```python
from build123d import *

# Parameters (mm, degrees)
F1_R     = 43.202069
F2_DEPTH = 60.706


with BuildPart() as f2:
    # F1 (on face) → F2 (new body)
    with BuildSketch(Plane.YZ):
        Circle(F1_R)
        Polygon((-6.760658, 25.522216), (22.183912, 14.316566), (20.471069, -16.674092), (-9.532095, -24.621722), (-26.362228, 1.457031), align=None, mode=Mode.SUBTRACT)
    extrude(amount=F2_DEPTH)


solid = f2.part
```
Source: CAD feature listing. Evaluate the final solid. Frame: model axes, mm. A direction names the side the tool comes from. Give positions to 0.01 mm unless a question says otherwise; leave off trailing zeros. Write each loop counter-clockwise with the first axis right and the second up, starting at its lowest first coordinate (ties: lowest second). Pieces come first, ordered by that corner, then holes.
1. Access query for faces 1 (the face through (29.928, 5.68, -20.592)), 2 (the face through (0, -20, -9)). Directions: +Z, -Z, +X, -X, +Y, -Y. A direction counts if a zero-diameter tool reaches every point of the face in a straight line with its end or side. Return the directions, or none.
2. Section query B-B (y = 16.5). Return the cut outline in (x, z).
3. Section query C-C (z = 0). Return the cut outline in (x, y).
4. Section query A-A (x = 22). Return the cut outline in (y, z), then the cut area to 3 significant figures.
5. Section query D-D (y = 28). Return the cut outline in (x, z), then the cut area to 3 significant figures.
6. Material intervals for line 1 along Z through (x, y) = (7, -14.5); line 2 along Y through (x, z) = (14, -13); line 3 along Z through (x, y) = (40.5, -0.5), sorted ascending.
7. First-contact query: pin 1 (6 mm diameter, centred on y = -8, z = -17.5, fed in from +X); pin 2 (1 mm diameter, centred on x = 27.5, z = 27.5, fed in from -Y); pin 3 (5 mm diameter, centred on x = 27.5, y = 30.5, fed in from -Z); pin 4 (5 mm diameter, centred on x = 38.5, y = -19.5, fed in from -Z). Flat tips, straight axial feed; report the tip coordinate or a pass-through.
8. Pull-direction query (Y, two-part tool) for faces 3 (the face through (29.9, 7.5, 20)), 4 (the face through (29.928, -9.365, -42.175)), 5 (the face through (60.706, -20, -9)); classes: +Y half, -Y half, draft (parallel to the pull), parting line (faces both ways), or undercut.
Output values:
1. face 1: +X, -X
1. face 2: +Z, -Z, -X, +Y, -Y
2. outline: (0, -39.93) - (60.71, -39.93) - (60.71, -17.73) - (0, -17.73) - close; (0, 16.52) - (60.71, 16.52) - (60.71, 39.93) - (0, 39.93) - close
3. outline: (0, -43.2) - (60.71, -43.2) - (60.71, -25.42) - (0, -25.42) - close; (0, 21.39) - (60.71, 21.39) - (60.71, 43.2) - (0, 43.2) - close
4. outline: circle Ø86.4 at (0, 0); hole (-26.36, 1.46) - (-9.53, -24.62) - (20.47, -16.67) - (22.18, 14.32) - (-6.76, 25.52) - close
4. area: 4,210 mm2
5. outline: (0, -32.9) - (60.71, -32.9) - (60.71, 32.9) - (0, 32.9) - close
5. area: 3,990 mm2
6. line 1: z = -40.7 to -16.92, 16.02 to 40.7
6. line 2: y = -41.2 to -17.03, 20.67 to 41.2
6. line 3: z = -43.2 to -22.23, 23.1 to 43.2
7. pin 1: passes through
7. pin 2: stops at y = -33.73
7. pin 3: stops at z = -32.9
7. pin 4: stops at z = -39.72
8. face 3: undercut
8. face 4: parting line
8. face 5: draft
